from build123d import *

# Parameters (mm, degrees)
SKETCH045_W     = 110
SKETCH045_H     = 32.6
PAD025_DEPTH    = 15.35
SKETCH046_W     = 9
SKETCH046_H     = 24.35
SKETCH046_R     = 2.25
PAD026_DEPTH    = 5
FILLET018_R     = 3.5
SKETCH047_W     = 101.4
SKETCH047_H     = 30.1
POCKET021_DEPTH = 10.35
SKETCH048_W     = 97
SKETCH048_H     = 2.5
POCKET022_DEPTH = 7.85
FILLET019_R     = 2
SKETCH049_W     = 66
SKETCH049_H     = 16.3
POCKET023_DEPTH = 5
FILLET020_R     = 2
FILLET021_R     = 2


with BuildPart() as part:
    # Sketch045 → Pad025 (new body)
    with BuildSketch(Plane.XY):
        Rectangle(SKETCH045_W, SKETCH045_H)
    extrude(amount=PAD025_DEPTH)

    # Sketch046 (on Face1 of Pad025) → Pad026 (join)
    with BuildSketch(Plane(origin=(0, 16.3, 0), x_dir=(-1, 0, 0), z_dir=(0, 1, 0))):
        with Locations((-37.5, 3.175)):
            Rectangle(SKETCH046_W, SKETCH046_H)
        with Locations((-37.5, -4.5)):
            Circle(SKETCH046_R, mode=Mode.SUBTRACT)
        with Locations((37.5, 3.175)):
            Rectangle(SKETCH046_W, SKETCH046_H)
        with Locations((37.5, -4.5)):
            Circle(SKETCH046_R, mode=Mode.SUBTRACT)
    extrude(amount=PAD026_DEPTH)

    # Fillet018
    fillet018_edges = [part.edges().sort_by_distance(p)[0] for p in [
        (42, 18.8, -9),
        (33, 18.8, -9),
        (-33, 18.8, -9),
        (-42, 18.8, -9),
    ]]
    fillet(fillet018_edges, radius=FILLET018_R)

    # Sketch047 (on Face7 of Fillet018) → Pocket021 (cut)
    with BuildSketch(Plane(origin=(0, 0, 0), x_dir=(1, 0, 0), z_dir=(0, 0, -1))):
        with Locations((0, -1.25)):
            Rectangle(SKETCH047_W, SKETCH047_H)
    extrude(amount=-POCKET021_DEPTH, mode=Mode.SUBTRACT)

    # Sketch048 (on Face12 of Pocket021) → Pocket022 (cut)
    with BuildSketch(Plane(origin=(0, 0, 0), x_dir=(1, 0, 0), z_dir=(0, 0, -1))):
        with Locations((0, 15.05)):
            Rectangle(SKETCH048_W, SKETCH048_H)
    extrude(amount=-POCKET022_DEPTH, mode=Mode.SUBTRACT)

    # Fillet019
    fillet019_edges = [part.edges().sort_by_distance(p)[0] for p in [
        (-48.5, -15.05, 7.85),
        (48.5, -15.05, 7.85),
    ]]
    fillet(fillet019_edges, radius=FILLET019_R)

    # Sketch049 (on Face20 of Fillet019) → Pocket023 (cut)
    with BuildSketch(Plane.XY.offset(15.35)):
        with Locations((0, 8.15)):
            Rectangle(SKETCH049_W, SKETCH049_H)
    extrude(amount=-POCKET023_DEPTH, mode=Mode.SUBTRACT)

    # Fillet020
    fillet020_edges = [part.edges().sort_by_distance(p)[0] for p in [
        (-33, 0, 12.85),
        (33, 0, 12.85),
        (-37.5, 16.3, 10.35),
        (37.5, 16.3, 10.35),
        (37.5, 21.3, 15.35),
        (-37.5, 21.3, 15.35),
    ]]
    fillet(fillet020_edges, radius=FILLET020_R)

    # Fillet021
    fillet021_edges = [part.edges().sort_by_distance(p)[0] for p in [
        (42, 16.3, 12.85),
        (-42, 16.3, 12.85),
    ]]
    fillet(fillet021_edges, radius=FILLET021_R)


with BuildPart() as part_1:
    # Body011 placement: moved
    add(part.part.moved(Location((0, 0, 51.75))))


solid = part_1.part
Source: CAD feature listing. Evaluate the final solid. Frame: model axes, mm. A direction names the side the tool comes from. Give positions to 0.01 mm unless a question says otherwise; leave off trailing zeros. Order: outer loops, then holes, each group sorted by start corner. A loop starts at its lowest first (then second) coordinate and runs counter-clockwise, first axis right, second up. Notation, with made-up numbers: (62, -34) -> (115, -34) arc R10 cw to (115, -16) -> close; hole circle Ø8 at (45.5, 28.25). An arc over 180 degrees is marked (long way). Use a Markdown table: item, result.
1) Mould query, pull axis Z, two halves, no side actions, for faces 6 (the flat face through (38, 19, 42.75)), 7 (the cylindrical face through (-37.56, 20.73, 66.5)), 8 (the cylindrical face through (32.4, 0.57, 64.56)), 9 (the cylindrical face through (-37.21, 18.76, 49.48)). Classes: +Z half, -Z half, draft (parallel to the pull), parting line (faces both ways), or undercut.
Answer list:
| item | result |
|---|---|
| face 6 | -Z half |
| face 7 | +Z half |
| face 8 | draft |
| face 9 | undercut |
2) Section query B-B, the plane y = 11. Return the cut outline in (x, z).
Answer list:
| item | result |
|---|---|
| outline | (-55, 51.75) -> (-50.7, 51.75) -> (-50.7, 62.1) -> (-33, 62.1) -> (-33, 67.1) -> (-55, 67.1) -> close; (33, 62.1) -> (50.7, 62.1) -> (50.7, 51.75) -> (55, 51.75) -> (55, 67.1) -> (33, 67.1) -> close |
3) Section query A-A, the plane x = 37.5. Return the cut outline in (y, z).
Answer list:
| item | result |
|---|---|
| outline | (-16.3, 59.6) -> (-13.8, 59.6) -> (-13.8, 62.1) -> (14.3, 62.1) arc R2 cw to (16.3, 60.1) -> (16.3, 49.5) -> (21.3, 49.5) -> (21.3, 65.1) arc R2 ccw to (19.3, 67.1) -> (-16.3, 67.1) -> close; (16.3, 42.75) -> (21.3, 42.75) -> (21.3, 45) -> (16.3, 45) -> close |
4) Section query C-C, the plane z = 47.25. Return the cut outline in (x, y).
Answer list:
| item | result |
|---|---|
| outline | (-42, 16.3) -> (-39.75, 16.3) -> (-39.75, 21.3) -> (-42, 21.3) -> close; (-35.25, 16.3) -> (-33, 16.3) -> (-33, 21.3) -> (-35.25, 21.3) -> close; (33, 16.3) -> (35.25, 16.3) -> (35.25, 21.3) -> (33, 21.3) -> close; (39.75, 16.3) -> (42, 16.3) -> (42, 21.3) -> (39.75, 21.3) -> close |
5) Contact query for flat-ended pins moving along their axis: P1, Ø7, axis at x = -37.5, z = 47.25, coming from the -Y side; P2, Ø7, axis at x = 53, y = 7.5, coming from the -Z side; P3, Ø3.5, axis at x = -51.5, z = 59, coming from the +Y side. Output: stop coordinate, or through.
Answer list:
| item | result |
|---|---|
| P1 | y = 16.3 |
| P2 | z = 51.75 |
| P3 | y = 16.3 |
6) Reachability of faces 1 (the cylindrical face through (-34, 18.8, 43.8)), 2 (the flat face through (-1, -15, 59.6)), 3 (the flat face through (0, 0, 65)), 4 (the flat face through (-51, 16.3, 61)), 5 (the cylindrical face through (41, 18.8, 43.8)) from +Z, -Z, +X, -X, +Y, -Y: full face, straight path, thin tool, end or side. Return the list, or none.
Answer list:
| item | result |
|---|---|
| face 1 | -Z, +Y, -Y |
| face 2 | -Z, -Y |
| face 3 | +Z, -Z, +Y |
| face 4 | +Z, -Z, -X, +Y |
| face 5 | -Z, +X, +Y, -Y |
7) Ray query, line 1 along X through (y, z) = (18, 46.5); line 2 along Z through (x, y) = (-37.5, 19.4); line 3 along X through (y, z) = (8, 59.5). Return the intervals inside material, ascending. Write a range as [from, to].
Answer list:
| item | result |
|---|---|
| line 1 | [-42, -39.62], [-35.38, -33], [33, 35.38], [39.62, 42] |
| line 2 | [42.75, 45], [49.5, 67.1] |
| line 3 | [-55, -50.7], [50.7, 55] |
8) Section query D-D, the plane z = 54.5. Return the cut outline in (x, y).
Answer list:
| item | result |
|---|---|
| outline | (-55, -16.3) -> (-48.5, -16.3) -> (-48.5, -13.8) -> (-50.7, -13.8) -> (-50.7, 16.3) -> (-55, 16.3) -> close; (-42, 16.3) -> (-33, 16.3) -> (-33, 21.3) -> (-42, 21.3) -> close; (33, 16.3) -> (42, 16.3) -> (42, 21.3) -> (33, 21.3) -> close; (48.5, -16.3) -> (55, -16.3) -> (55, 16.3) -> (50.7, 16.3) -> (50.7, -13.8) -> (48.5, -13.8) -> close |
